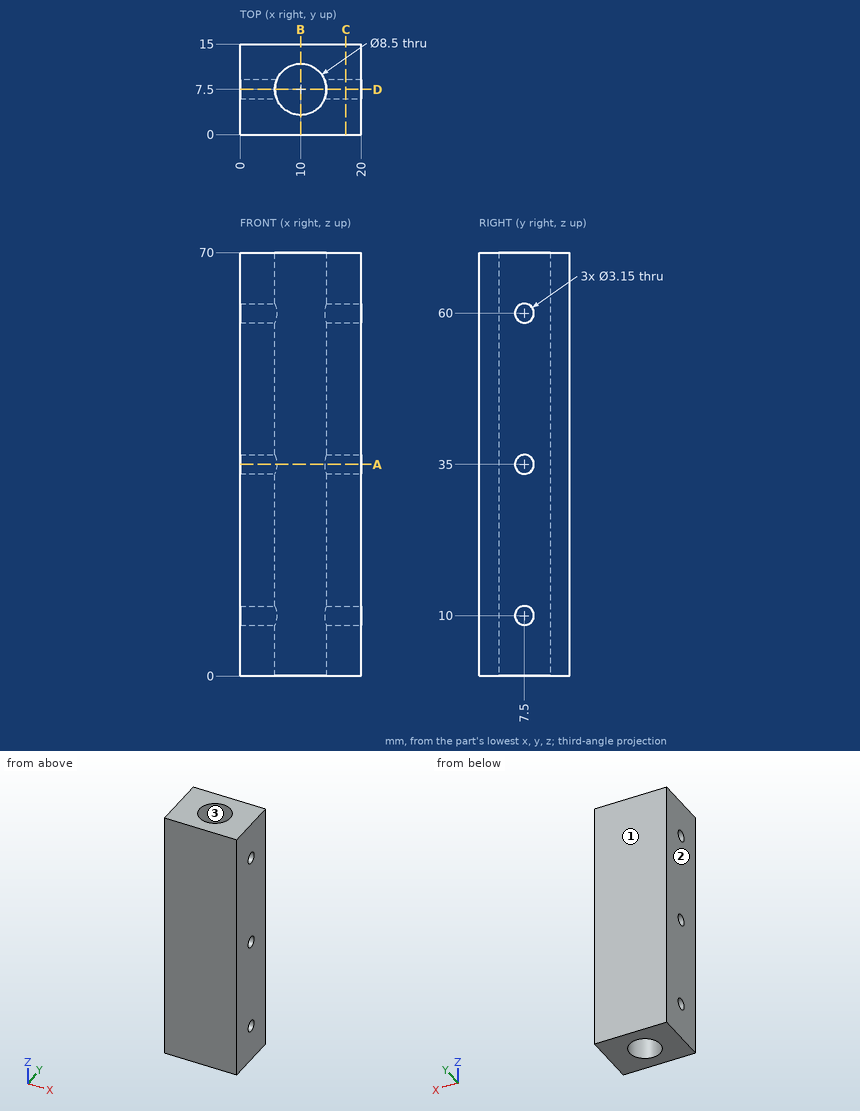
Can you work these out from the drawing? Everything is in mm from the part's minimum corner. Coordinates: 2 decimals unless noted, no trailing zeros. Write each loop counter-clockwise with the first axis right and the second up, starting at its lowest first coordinate (ties: lowest second). Pieces come first, ordered by that corner, then holes. Notation, with made-up numbers: (86.25, -2.5) - (133.25, -2.5) arc R38 ccw to (133.25, 35.5) - close; hole circle Ø3 at (21.25, 2). An arc over 180 degrees is marked (long way). Use a Markdown table: item, result.
Q1. Imagine slicing it at D-D (y = 7.5). Count the separate pieces of the cut face and the enclosed holes in it, and give its area (3 significant figures).
Geometry check:
| item | result |
|---|---|
| separate pieces | 8 |
| enclosed holes | 0 |
| area | 696 mm2 |
Q2. Thinking about a two-plate mould opening in Y: for the marked faces 1, 2 and 3, which applies, +Y half, -Y half, draft (parallel to the pull), parting line (faces both ways), or undercut?
Geometry check:
| item | result |
|---|---|
| face 1 | +Y half |
| face 2 | draft |
| face 3 | undercut |
Q3. Please list where these lines run through material, in increasing order: L1, parallel to Z at x = 2, y = 7.5 (3 decimals); L2, parallel to Y at x = 10, z = 19; L3, parallel to X at y = 7.25, z = 12.5.
Geometry check:
| item | result |
|---|---|
| L1 | z = 0 to 8.425, 11.575 to 33.425, 36.575 to 58.425, 61.575 to 70 |
| L2 | y = 0 to 3.25, 11.75 to 15 |
| L3 | x = 0 to 5.76, 14.24 to 20 |
Q4. Imagine slicing it at A-A (z = 35). List the corners of the cut face in (x, y) for me (3 decimals), and give its area (3 significant figures).
Geometry check:
| item | result |
|---|---|
| outline | (0, 0) - (20, 0) - (20, 5.925) - (13.947, 5.925) arc R4.25 cw to (6.053, 5.925) - (0, 5.925) - close; (0, 9.075) - (6.053, 9.075) arc R4.25 cw to (13.947, 9.075) - (20, 9.075) - (20, 15) - (0, 15) - close |
| area | 206 mm2 |
Q5. Imagine slicing it at C-C (x = 17.5). List the corners of the cut face in (y, z) for me (3 decimals), and give its area (3 significant figures).
Geometry check:
| item | result |
|---|---|
| outline | (0, 0) - (15, 0) - (15, 70) - (0, 70) - close; hole circle Ø3.15 at (7.5, 10); hole circle Ø3.15 at (7.5, 35); hole circle Ø3.15 at (7.5, 60) |
| area | 1,030 mm2 |
Q6. Imagine slicing it at B-B (x = 10). List the corners of the cut face in (y, z) for me, and give its area (3 significant figures).
Geometry check:
| item | result |
|---|---|
| outline | (0, 0) - (3.25, 0) - (3.25, 70) - (0, 70) - close; (11.75, 0) - (15, 0) - (15, 70) - (11.75, 70) - close |
| area | 455 mm2 |
